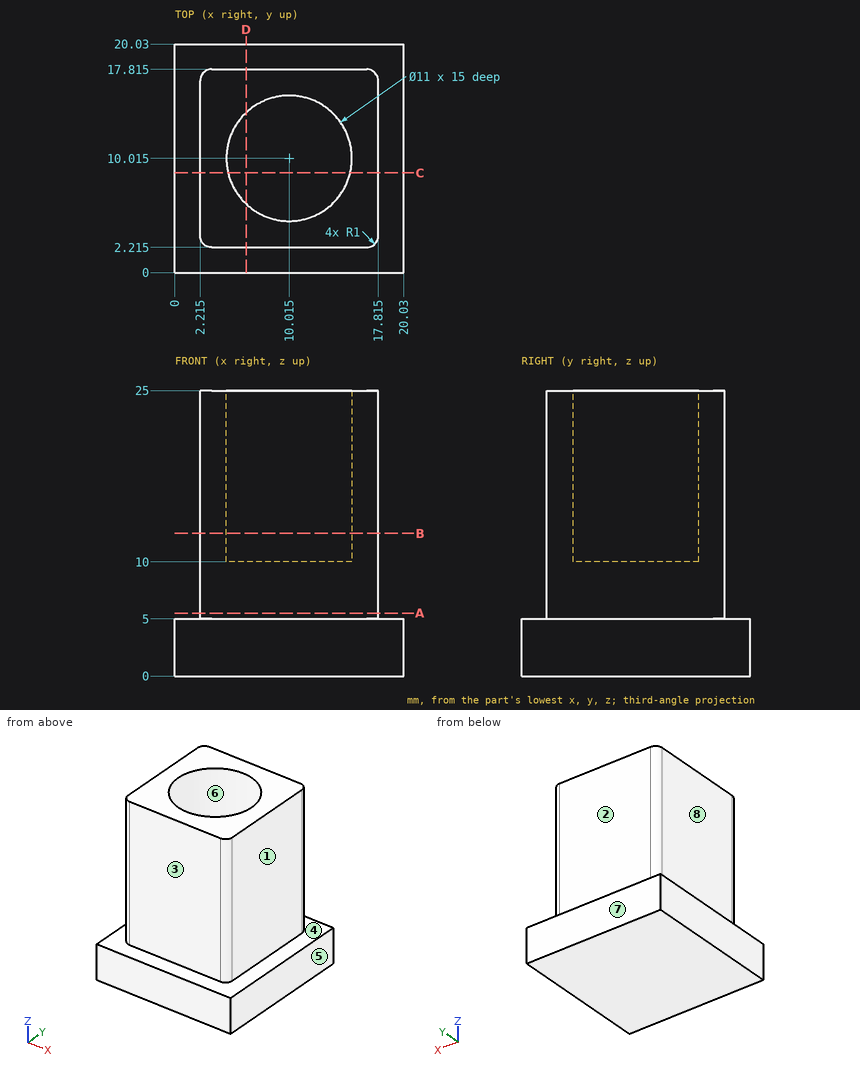
Part print with two shaded views. Sizes in mm from the minimum x, y, z corner. A direction names the side the tool comes from. Coordinates: 2 decimals unless noted, no trailing zeros. Write each loop counter-clockwise with the first axis right and the second up, starting at its lowest first coordinate (ties: lowest second). Pieces come first, ordered by that corner, then holes. Notation, with made-up numbers: (77, -9) -> (113, -9) arc R18 ccw to (113, -1) -> close; hole circle Ø10 at (58.25, 80). An arc over 180 degrees is marked (long way). Return JSON: item names as keys, results as strings. Group by question number.
Q1. Pull direction X, two halves, no side cores. Call the marked faces 5, 6, 7 and 8: released by +X, released by -X, zero draft, split by the parting line, or undercut.
Q2. Cut at D-D, the plane x = 6.25. Give the cut face in (y, z) (3 decimals), then the cut area to 3 significant figures.
Q3. Drill centre lines: line 1 (X direction, y = 5.25, z = 7.75) (3 decimals); line 2 (Z direction, x = 18.25, y = 15.5); line 3 (X direction, y = 5.5, z = 19.75) (3 decimals). Where is each one in solid material? Low to high.
Q4. Cut at A-A, the plane z = 5.5. Give the cut face in (x, y) (3 decimals), then the cut area to 3 significant figures.
Q5. Cut at C-C, the plane y = 8.75. Give the cut face in (x, z) (3 decimals).
Q6. Cut at B-B, the plane z = 12.5. Give the cut face in (x, y) (3 decimals).
Q7. Flat gauge pins, fed straight in: pin 1 (7 mm diameter, centred on y = 10.5, z = 14, fed in from +X) (3 decimals); pin 2 (4 mm diameter, centred on y = 9.5, z = 17, fed in from -X) (3 decimals); pin 3 (7 mm diameter, centred on x = 12, z = 14, fed in from +Y) (3 decimals). Where does each tip first touch, or does it go through?
Q8. Which spindle directions (+Z, -Z, +X, -X, +Y, -Y) get a long thin tool onto all of the face, cutting with end or side? Do the marked faces 1, 2, 3 and 4. Say none if no direction does.
Returned:
{
 "1": {"face 5": "released by +X", "face 6": "undercut", "face 7": "zero draft", "face 8": "released by -X"},
 "2": {"outline": "(0, 0) -> (20.03, 0) -> (20.03, 5) -> (17.815, 5) -> (17.815, 25) -> (14.024, 25) -> (14.024, 10) -> (6.006, 10) -> (6.006, 25) -> (2.215, 25) -> (2.215, 5) -> (0, 5) -> close", "area": "292 mm2"},
 "3": {"line 1": "x = 2.215 to 17.815", "line 2": "z = 0 to 5", "line 3": "x = 2.215 to 6.874, 13.156 to 17.815"},
 "4": {"outline": "(2.215, 3.215) arc R1 ccw to (3.215, 2.215) -> (16.815, 2.215) arc R1 ccw to (17.815, 3.215) -> (17.815, 16.815) arc R1 ccw to (16.815, 17.815) -> (3.215, 17.815) arc R1 ccw to (2.215, 16.815) -> close", "area": "243 mm2"},
 "5": {"outline": "(0, 0) -> (20.03, 0) -> (20.03, 5) -> (17.815, 5) -> (17.815, 25) -> (15.368, 25) -> (15.368, 10) -> (4.662, 10) -> (4.662, 25) -> (2.215, 25) -> (2.215, 5) -> (0, 5) -> close"},
 "6": {"outline": "(2.215, 3.215) arc R1 ccw to (3.215, 2.215) -> (16.815, 2.215) arc R1 ccw to (17.815, 3.215) -> (17.815, 16.815) arc R1 ccw to (16.815, 17.815) -> (3.215, 17.815) arc R1 ccw to (2.215, 16.815) -> close; hole circle Ø11 at (10.015, 10.015)"},
 "7": {"pin 1": "stops at x = 17.815", "pin 2": "stops at x = 2.215", "pin 3": "stops at y = 17.815"},
 "8": {"face 1": "+Z, +X, +Y, -Y", "face 2": "+Z, +X, -X, +Y", "face 3": "+Z, +X, -X, -Y", "face 4": "+Z"}
}
